Verification items for this drawing (mm, ordinates from the low corner). A direction names the side the tool comes from. Give positions to 0.01 mm unless a question says otherwise; leave off trailing zeros. Order: outer loops, then holes, each group sorted by start corner. A loop starts at its lowest first (then second) coordinate and runs counter-clockwise, first axis right, second up. Notation, with made-up numbers: (3, -31) - (59, -31) arc R9 ccw to (59, -18) - close; hole circle Ø7 at (26, 68). An arc over 180 degrees is marked (long way). Put each result on its own line as item: value. Start each with the question number.
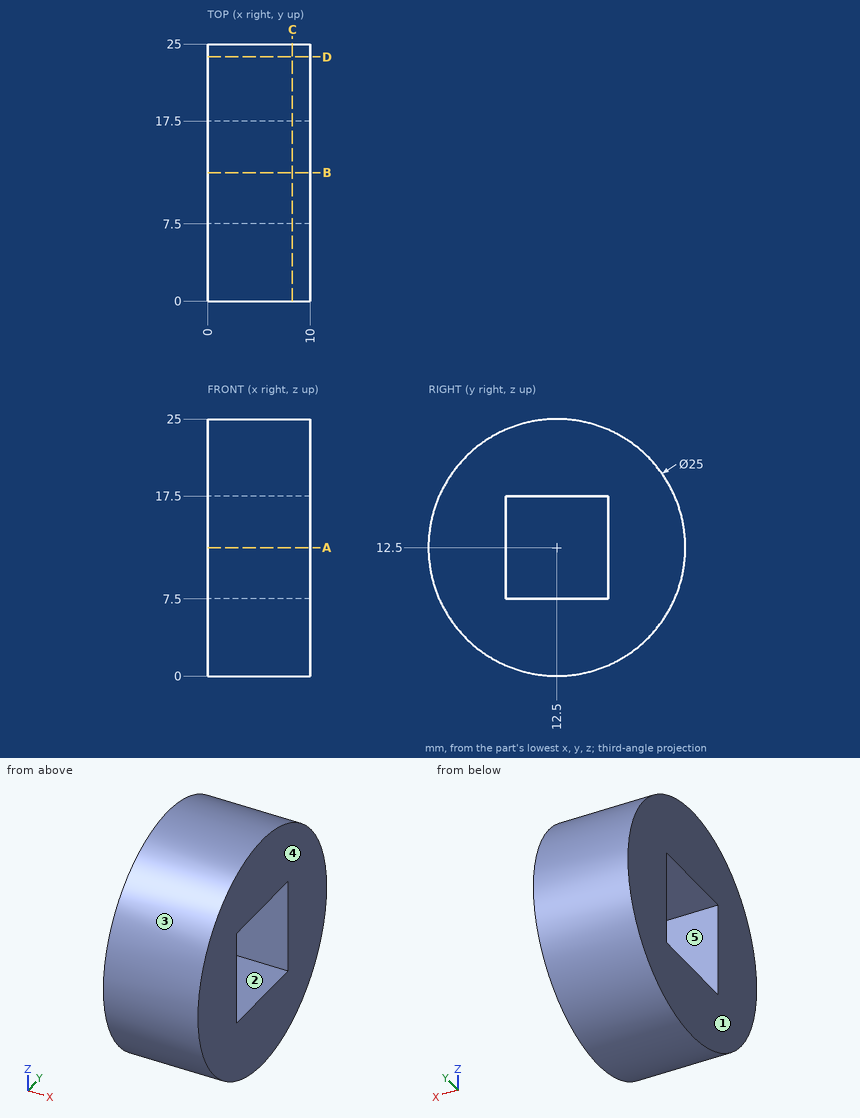
Item 1: Cross-section at A-A (z = 12.5). Enter the section's corners in (x, y).
Item 2: Thickness scan on line 1 along Z through (x, y) = (1.5, 11.75); line 2 along Z through (x, y) = (5.25, 16.5); line 3 along Y through (x, z) = (4.5, 15). Record the ranges inside material, lowest first.
Item 3: Cross-section at D-D (y = 23.75). Enter the section's corners in (x, z).
Item 4: Release check for a two-part mould opening along Z. For the marked faces 3, 4 and 5 record: +Z half, -Z half, draft (parallel to the pull), parting line (faces both ways), or undercut.
Item 5: Cross-section at C-C (x = 8.25). Enter the section's corners in (y, z).
Item 6: Set-up check for the marked faces 1 and 2: record each of +Z, -Z, +X, -X, +Y, -Y from which the full face is reachable in a straight line by a thin tool's end or side.
Item 7: Gauge pin test, flat ends, axial feed: pin 1 Ø6 at (x, z) = (6, 19.5) entering from +Y; pin 2 Ø1 at (x, y) = (8.5, 7) entering from -Z; pin 3 Ø6 at (x, z) = (7, 22.5) entering from -Y; pin 4 Ø3 at (x, z) = (2.5, 14) entering from -Y. Record the tip position at first contact, or that the pin passes through.
Recorded:
1. outline: (0, 0) - (10, 0) - (10, 7.5) - (0, 7.5) - close; (0, 17.5) - (10, 17.5) - (10, 25) - (0, 25) - close
2. line 1: z = 0.02 to 7.5, 17.5 to 24.98
2. line 2: z = 0.66 to 7.5, 17.5 to 24.34
2. line 3: y = 0.25 to 7.5, 17.5 to 24.75
3. outline: (0, 7.05) - (10, 7.05) - (10, 17.95) - (0, 17.95) - close
4. face 3: parting line
4. face 4: draft
4. face 5: undercut
5. outline: circle Ø25 at (12.5, 12.5); hole (7.5, 7.5) - (17.5, 7.5) - (17.5, 17.5) - (7.5, 17.5) - close
6. face 1: +Z, -Z, -X, +Y, -Y
6. face 2: +X, -X
7. pin 1: stops at y = 24.34
7. pin 2: stops at z = 1.04
7. pin 3: stops at y = 2.14
7. pin 4: stops at y = 0
